Read the model definition and answer for the solid it produces. Units are mm, in the model's axes. Face numbers are marked on the shaded views. A direction names the side the tool comes from. Give positions to 0.01 mm unless a question says otherwise; leave off trailing zeros. Write each loop counter-clockwise with the first axis right and the second up, starting at its lowest first coordinate (ties: lowest second). Pieces come first, ordered by that corner, then holes. Notation, with made-up numbers: (0, -17) -> (36, -17) arc R17 cw to (36, -11) -> close; hole circle Ø9 at (0.25, 84.5). An arc over 180 degrees is marked (long way). Use a Markdown table: item, result.
from build123d import *

# Parameters (mm, degrees)
SKETCH1_R                = 74.295
BOSS_EXTRUDE1_DEPTH      = 46.228
FILLET1_R                = 6.35
SKETCH2_R                = 4.445
BOSS_EXTRUDE2_DEPTH      = 19.05
BOSS_EXTRUDE2_DEPTH_BACK = 65.278


with BuildPart() as part:
    # Sketch1 → Boss-Extrude1 (new body)
    with BuildSketch(Plane.XY):
        Circle(SKETCH1_R)
    extrude(amount=BOSS_EXTRUDE1_DEPTH)

    # Fillet1
    fillet1_edges = [part.edges().sort_by_distance(p)[0] for p in [
        (-74.295, 0, 0),
        (-74.295, 0, 46.228),
    ]]
    fillet(fillet1_edges, radius=FILLET1_R)

    # Sketch2 → Boss-Extrude2 (add, two sides)
    with BuildSketch(Plane.XY.offset(46.228)) as boss_extrude2_sk:
        Circle(SKETCH2_R)
    extrude(amount=BOSS_EXTRUDE2_DEPTH)
    extrude(boss_extrude2_sk.sketch, amount=-BOSS_EXTRUDE2_DEPTH_BACK)


solid = part.part
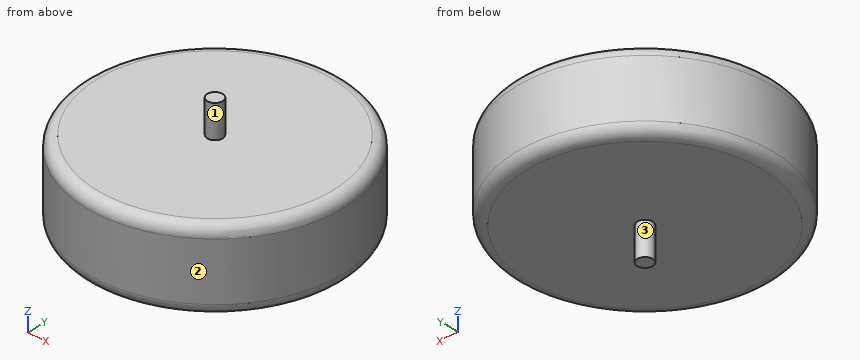
Item 1: Straight lines are drawn through the part: line 1 along Y through (x, z) = (30, 21); line 2 along Z through (x, y) = (27, -3); line 3 along X through (y, z) = (2, 59). For each, find the intervals that lie inside material, in ascending order. Write a range as [from, to].
Return value:
| item | result |
|---|---|
| line 1 | [-67.97, 67.97] |
| line 2 | [0, 46.23] |
| line 3 | [-3.97, 3.97] |
Item 2: Each of these flat-tipped pins is pushed along its axis until it touches: P1, Ø2, axis at y = -46.5, z = 11.5, coming from the +X side; P2, Ø6, axis at x = -58, y = 22, coming from the +Z side; P3, Ø4, axis at y = 38, z = 29, coming from the -X side; P4, Ø12, axis at y = 41, z = 53.5, coming from the +X side. Where does it stop, or does it pass through?
Return value:
| item | result |
|---|---|
| P1 | x = 58.73 |
| P2 | z = 46.23 |
| P3 | x = -64.99 |
| P4 | through |
Item 3: A cutting plane is placed at C-C (z = 12). Give the vertices of the cut face in (x, y) (3 decimals), then the cut area to 3 significant figures.
Return value:
| item | result |
|---|---|
| outline | circle Ø148.59 at (0, 0) |
| area | 17,300 mm^2 |
Item 4: A tool of negligible diameter and unlimited length cuts with its end or side. For the marked faces 1, 2 and 3, from which of +Z, -Z, +X, -X, +Y, -Y can it reach the whole face along a straight path? Write none if from no direction.
Return value:
| item | result |
|---|---|
| face 1 | +Z |
| face 2 | +Z, -Z |
| face 3 | -Z |
Item 5: A cutting plane is placed at D-D (z = 52). Give the vertices of the cut face in (x, y) (3 decimals).
Return value:
| item | result |
|---|---|
| outline | circle Ø8.89 at (0, 0) |
Item 6: A cutting plane is placed at A-A (y = 0). Give the vertices of the cut face in (x, z) (3 decimals), then the cut area to 3 significant figures.
Return value:
| item | result |
|---|---|
| outline | (-74.295, 6.35) arc R6.35 ccw to (-67.945, 0) -> (-4.445, 0) -> (-4.445, -19.05) -> (4.445, -19.05) -> (4.445, 0) -> (67.945, 0) arc R6.35 ccw to (74.295, 6.35) -> (74.295, 39.878) arc R6.35 ccw to (67.945, 46.228) -> (4.445, 46.228) -> (4.445, 65.278) -> (-4.445, 65.278) -> (-4.445, 46.228) -> (-67.945, 46.228) arc R6.35 ccw to (-74.295, 39.878) -> close |
| area | 7,170 mm^2 |
